The listing builds one solid part. Answer for the finished solid, in the listing's coordinates (mm). A direction names the side the tool comes from. Give positions to 0.01 mm unless a question says otherwise; leave off trailing zeros. Write each loop counter-clockwise with the first axis right and the second up, starting at its lowest first coordinate (ties: lowest second). Pieces come first, ordered by that corner, then holes. Notation, with made-up numbers: (78, 60.25) -> (102, 60.25) arc R34 cw to (102, 96.25) -> close; hole circle Ø7 at (36.5, -20). An arc over 180 degrees is marked (long way). Put each result on its own line as item: value. Start each with the question number.
1) For a pull along Y with two mould halves and no side action, classify faces 3 (the flat face through (221.5, 15.7, -1.6)), 4 (the flat face through (3, -52, -7)), 5 (the flat face through (-3, 1, -2)), 6 (the flat face through (-3, 52, -15)) as released by +Y, released by -Y, zero draft, split by the parting line, or undercut.
2) A cutting plane is placed at A-A (x = 188.5). Write down the section's boundary in (y, z).
3) Flat-ended cylindrical pins translate along their axes: pin 1 Ø2 at (x, y) = (-24.5, -50.5) entering from -Z; pin 2 Ø8 at (y, z) = (-21, -9) entering from -X; pin 3 Ø1.5 at (x, y) = (51, -6.5) entering from +Z; pin 4 Ø10 at (x, y) = (-117.5, -35) entering from -Z. Find the tip coordinate at first contact, or state that the pin passes through.
4) A cutting plane is placed at B-B (y = 9). Write down the section's boundary in (x, z), then the cut area to 3 significant figures.
5) Find the intervals of material crossed by line 1 along Y through (x, z) = (65.5, -10.5); line 2 along Y through (x, z) = (-147, -24.5); line 3 along Z through (x, y) = (118, -0.5), in increasing order. Write a range as from..to.
6) For faces 1 (the flat face through (-3, 50, -15)), 2 (the flat face through (-221.5, 15.7, -1.6)), determine the directions among +Z, -Z, +X, -X, +Y, -Y from which every point of the face is accessible in a straight line to the end or side of a thin tool.
from build123d import *

# Parameters (mm, degrees)
SKETCH1_W                    = 443
SKETCH1_H                    = 100
BASE_FLANGE1_DEPTH           = 2
EDGE_FLANGE1_STRIP_W         = 10
EDGE_FLANGE1_STRIP_H         = 2
EDGE_FLANGE1_STRIP_CUT_DEPTH = 443
EDGE_FLANGE1_DEPTH           = 443
EDGE_FLANGE2_STRIP_W         = 10
EDGE_FLANGE2_STRIP_H         = 2
EDGE_FLANGE2_STRIP_CUT_DEPTH = 443
EDGE_FLANGE2_DEPTH           = 443
CUT_EXTRUDE2_DEPTH           = 10


# Sheet-metal steps are written as plain solids
with BuildPart() as part:
    # Sketch1 → Base-Flange1 (new body)
    with BuildSketch(Plane.XY):
        Rectangle(SKETCH1_W, SKETCH1_H)
    extrude(amount=-BASE_FLANGE1_DEPTH)

    # Edge-Flange1 strip (across the edge) → Edge-Flange1 strip cut (cut)
    with BuildSketch(Plane(origin=(-221.5, 50, -2), x_dir=(0, -1, 0), z_dir=(1, 0, 0))):
        with Locations((-4, -1)):
            Rectangle(EDGE_FLANGE1_STRIP_W, EDGE_FLANGE1_STRIP_H)
    extrude(amount=EDGE_FLANGE1_STRIP_CUT_DEPTH, mode=Mode.SUBTRACT)

    # Edge-Flange1 section (across the edge) → Edge-Flange1 (add)
    with BuildSketch(Plane(origin=(-221.5, 50, -2), x_dir=(0, -1, 0), z_dir=(1, 0, 0))):
        with BuildLine():
            Line((-2, 1), (-2, 25))
            Line((-2, 25), (0, 25))
            Line((0, 25), (0, 1))
            ThreePointArc((0, 1), (0.292893219, 0.292893219), (1, 0))
            Line((1, 0), (1, -2))
            ThreePointArc((1, -2), (-1.121320344, -1.121320344), (-2, 1))
        make_face()
    extrude(amount=EDGE_FLANGE1_DEPTH)

    # Edge-Flange2 strip (across the edge) → Edge-Flange2 strip cut (cut)
    with BuildSketch(Plane(origin=(221.5, -50, -2), x_dir=(0, 1, 0), z_dir=(-1, 0, 0))):
        with Locations((-4, -1)):
            Rectangle(EDGE_FLANGE2_STRIP_W, EDGE_FLANGE2_STRIP_H)
    extrude(amount=EDGE_FLANGE2_STRIP_CUT_DEPTH, mode=Mode.SUBTRACT)

    # Edge-Flange2 section (across the edge) → Edge-Flange2 (add)
    with BuildSketch(Plane(origin=(221.5, -50, -2), x_dir=(0, 1, 0), z_dir=(-1, 0, 0))):
        with BuildLine():
            Line((-2, 1), (-2, 10))
            Line((-2, 10), (0, 10))
            Line((0, 10), (0, 1))
            ThreePointArc((0, 1), (0.292893219, 0.292893219), (1, 0))
            Line((1, 0), (1, -2))
            ThreePointArc((1, -2), (-1.121320344, -1.121320344), (-2, 1))
        make_face()
    extrude(amount=EDGE_FLANGE2_DEPTH)

    # Sketch13 → Cut-Extrude2 (cut)
    with BuildSketch(Plane(origin=(0, 52, 0), x_dir=(1, 0, 0), z_dir=(0, 1, 0))):
        with BuildLine():
            ThreePointArc((0, 24.5), (-2.5, 22), (0, 19.5))
            Line((0, 19.5), (0, 24.5))
        make_face()
        with BuildLine():
            Line((0, 24.5), (0, 19.5))
            ThreePointArc((0, 19.5), (1.767766953, 20.232233047), (2.5, 22))
            ThreePointArc((2.5, 22), (1.767766953, 23.767766953), (0, 24.5))
        make_face()
    extrude(amount=-CUT_EXTRUDE2_DEPTH, mode=Mode.SUBTRACT)


solid = part.part
Reply:
1. face 3: zero draft
1. face 4: released by -Y
1. face 5: undercut
1. face 6: released by +Y
2. outline: (-52, -12) -> (-50, -12) -> (-50, -3) arc R1 cw to (-49, -2) -> (49, -2) arc R1 cw to (50, -3) -> (50, -27) -> (52, -27) -> (52, -3) arc R3 ccw to (49, 0) -> (-49, 0) arc R3 ccw to (-52, -3) -> close
3. pin 1: stops at z = -12
3. pin 2: passes through
3. pin 3: stops at z = 0
3. pin 4: stops at z = -2
4. outline: (-221.5, -2) -> (221.5, -2) -> (221.5, 0) -> (-221.5, 0) -> close
4. area: 886 mm2
5. line 1: y = -52..-50, 50..52
5. line 2: y = 50..52
5. line 3: z = -2..0
6. face 1: -Z, +X, -X
6. face 2: +Z, -Z, -X, +Y, -Y
